Geometry check sheet. Reference: the model listing, model coordinates, mm. Face numbers are marked on the shaded views. A direction names the side the tool comes from. Round coordinates to 2 decimals unless told otherwise and drop trailing zeros. Order: outer loops, then holes, each group sorted by start corner. A loop starts at its lowest first (then second) coordinate and runs counter-clockwise, first axis right, second up. Notation, with made-up numbers: (58.5, -13) - (81.5, -13) arc R34 cw to (81.5, 17) - close; hole circle Ø5 at (-7.75, 2). An arc over 180 degrees is marked (long way). Write each question's results on one line, items separated by ' | '.
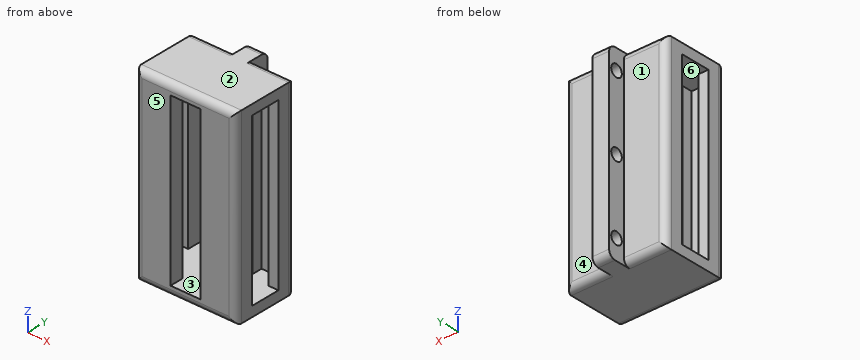
```python
from build123d import *

# Parameters (mm, degrees)
BOSS_EXTRUDE1_DEPTH = 28
CUT_EXTRUDE3_START  = -1.5
CUT_EXTRUDE3_DEPTH  = 25
SKETCH3_R           = 0.9
CUT_EXTRUDE2_DEPTH  = 2.5
FILLET2_R           = 1


with BuildPart() as part:
    # Sketch1 → Boss-Extrude1 (new body)
    with BuildSketch(Plane.XY):
        Polygon((0, 0), (15, 0), (15, 10), (8.75, 10), (8.75, 12.5), (6.25, 12.5), (6.25, 10), (0, 10), align=None)
    extrude(amount=-BOSS_EXTRUDE1_DEPTH)

    # Sketch4 → Cut-Extrude3 (cut)
    with BuildSketch(Plane.XY.offset(CUT_EXTRUDE3_START)):
        Polygon((10.5, 8), (10.5, 9.5), (13.5, 9.5), (13.5, 7.25), (15, 7.25), (15, 2.75), (13.5, 2.75), (13.5, 0.5), (10.5, 0.5), (10.5, 2), (9.75, 2), (9.75, 0), (5.25, 0), (5.25, 2), (4.5, 2), (4.5, 0.5), (1.5, 0.5), (1.5, 2.75), (0, 2.75), (0, 7.25), (1.5, 7.25), (1.5, 9.5), (4.5, 9.5), (4.5, 8), align=None)
    extrude(amount=-CUT_EXTRUDE3_DEPTH, mode=Mode.SUBTRACT)

    # Sketch3 → Cut-Extrude2 (cut)
    with BuildSketch(Plane(origin=(8.75, 0, 0), x_dir=(0, 0, -1), z_dir=(1, 0, 0))):
        with Locations((14, 11.25)):
            Circle(SKETCH3_R)
        with Locations((3, 11.25)):
            Circle(SKETCH3_R)
        with Locations((25, 11.25)):
            Circle(SKETCH3_R)
    extrude(amount=-CUT_EXTRUDE2_DEPTH, mode=Mode.SUBTRACT)

    # Fillet2
    fillet2_edges = [part.edges().sort_by_distance(p)[0] for p in [
        (7.5, 0, 0),
        (11.875, 10, -28),
        (0, 10, -14),
        (15, 10, -14),
        (15, 0, -14),
        (0, 0, -14),
        (7.5, 12.5, -28),
        (3.125, 10, -28),
        (7.5, 0, -28),
        (3.125, 10, 0),
        (7.5, 12.5, 0),
        (11.875, 10, 0),
    ]]
    fillet(fillet2_edges, radius=FILLET2_R)


solid = part.part
```
(1) Section check A-A (x = 2.5). Record the cut outline in (y, z), then the cut area to 3 significant figures.
Answers follow:
outline: (0, -27) arc R1 ccw to (1, -28) - (9, -28) arc R1 ccw to (10, -27) - (10, -1) arc R1 ccw to (9, 0) - (1, 0) arc R1 ccw to (0, -1) - close; hole (0.5, -26.5) - (9.5, -26.5) - (9.5, -1.5) - (0.5, -1.5) - close | area: 54.1 mm²
(2) Section check B-B (y = 6). Record the cut outline in (x, z), then the cut area to 3 significant figures.
Answers follow:
outline: (0, -28) - (15, -28) - (15, -26.5) - (0, -26.5) - close; (0, -1.5) - (15, -1.5) - (15, 0) - (0, 0) - close | area: 45.0 mm²
(3) Section check C-C (z = -22.25). Give the number of separate pieces and of enclosed holes in the cut face, then the cut area to 3 significant figures.
Answers follow:
separate pieces: 3 | enclosed holes: 0 | area: 42.9 mm²
(4) Draft check along Y on the marked faces 3, 4, 5 and 6. Enter one of: released by +Y, released by -Y, zero draft, split by the parting line, or undercut.
Answers follow:
face 3: undercut | face 4: released by +Y | face 5: released by -Y | face 6: undercut
(5) Access from +Z, -Z, +X, -X, +Y, -Y to the whole of each face (thin tool, end or side, straight path). Record for the marked faces 1 and 2.
Answers follow:
face 1: +Z, -Z, -X, +Y | face 2: +Z, +X, -X, +Y, -Y
(6) Depth check by flat-ended pin: pin 1 Ø4 at (y, z) = (10.5, -12.5) entering from +X; pin 2 Ø1.6 at (x, z) = (1, -19.5) entering from +Y. Enter the tip coordinate at first touch or a pass-through.
Answers follow:
pin 1: x = 15 | pin 2: y = 10
(7) Material ranges on line 1 (X direction, y = 9, z = -4); line 2 (Y direction, x = 10.25, z = -25); line 3 (Y direction, x = 4, z = -12.5), recorded low to high.
Answers follow:
line 1: 0 to 1.5, 4.5 to 10.5, 13.5 to 15 | line 2: 0 to 2, 8 to 10 | line 3: 0 to 0.5, 9.5 to 10
